from build123d import *

# Parameters (mm, degrees)
SKETCH1_R          = 317.5
BASE_FLANGE1_DEPTH = 5
SKETCH8_R          = 77.5
CUT_EXTRUDE1_DEPTH = 10
SKETCH15_R         = 5
CUT_EXTRUDE2_DEPTH = 10
CIRPATTERN1_COUNT  = 9


# Sheet-metal steps are written as plain solids
with BuildPart() as part:
    # Sketch1 → Base-Flange1 (new body)
    with BuildSketch(Plane.XY):
        Circle(SKETCH1_R)
    extrude(amount=-BASE_FLANGE1_DEPTH)

    # Sketch8 → Cut-Extrude1 (cut)
    with BuildSketch(Plane(origin=(0, 0, -5), x_dir=(-1, 0, 0), z_dir=(0, 0, -1))):
        Circle(SKETCH8_R)
    extrude(amount=-CUT_EXTRUDE1_DEPTH, mode=Mode.SUBTRACT)

    # Sketch15 → Cut-Extrude2 (cut)
    with BuildSketch(Plane(origin=(0, 0, -5), x_dir=(-1, 0, 0), z_dir=(0, 0, -1))):
        with Locations((0, 92.5)):
            Circle(SKETCH15_R)
    cut_extrude2 = extrude(amount=-CUT_EXTRUDE2_DEPTH, mode=Mode.SUBTRACT)

    # CirPattern1: Cut-Extrude2 ×9 about axis
    cirpattern1_axis = Axis((0, 0, 0), (0, 0, 1))
    for i in range(1, CIRPATTERN1_COUNT):
        add(cut_extrude2.rotate(cirpattern1_axis, i * 360 / CIRPATTERN1_COUNT), mode=Mode.SUBTRACT)


solid = part.part
Here's how the part is built. I have some questions about the finished solid (model axes, mm). Round coordinates to 2 decimals unless told otherwise and drop trailing zeros. Loops run counter-clockwise (first coordinate to the right, second up) from the corner with the lowest first, then second, coordinate; pieces in that order, holes last.
1. For P1, Ø6, axis at x = -91.09, y = 16.06, coming from the -Z side; P2, Ø2, axis at x = -248.5, z = -1, coming from the +Y side; P3, Ø1.5, axis at x = -144.5, z = -2, coming from the +Y side, each with a flat end and sliding along its axis, tell me the tip position at first contact or that it passes through.
Answer list:
P1: passes through
P2: stops at y = 198.87
P3: stops at y = 283.09
2. If we section it at B-B on x = 115: Write out the boundary of the cut face in (y, z), plus the area to 3 significant figures.
Answer list:
outline: (-295.94, -5) - (295.94, -5) - (295.94, 0) - (-295.94, 0) - close
area: 2,960 mm2
3. If I drill on line 1 along Y through (x, z) = (0, -1.55); line 2 along Y through (x, z) = (30.5, -4.7); line 3 along Y through (x, z) = (-91, -3.85), over which ranges is the centre line in solid material (lowest first)?
Answer list:
line 1: y = -317.5 to -77.5, 77.5 to 87.5, 97.5 to 317.5
line 2: y = -316.03 to -91.79, -82.05 to -71.25, 71.25 to 316.03
line 3: y = -304.18 to 11.06, 21.06 to 304.18
4. If we section it at C-C on y = 241: Write out the boundary of the cut face in (x, z).
Answer list:
outline: (-206.7, -5) - (206.7, -5) - (206.7, 0) - (-206.7, 0) - close
5. We'd pull the mould along Y, two halves only. Please class faces 1 (the face through (16.8, -75.657, -2.535)), 2 (the face through (66, -66, 0)), 3 (the face through (302.84, 95.37, -2.46)): +Y half, -Y half, draft (parallel to the pull), parting line (faces both ways), or undercut.
Answer list:
face 1: undercut
face 2: draft
face 3: parting line
6. If we section it at A-A on z = -3.1: Count the separate pieces of the cut face and the enclosed holes in it, plus the area to 3 significant figures.
Answer list:
separate pieces: 1
enclosed holes: 10
area: 297,000 mm2
